Here's the drawing with two shaded views (mm, measured from the low corner). I have some questions. A direction names the side the tool comes from. Give positions to 0.01 mm unless a question says otherwise; leave off trailing zeros. Order: outer loops, then holes, each group sorted by start corner. A loop starts at its lowest first (then second) coordinate and runs counter-clockwise, first axis right, second up. Notation, with made-up numbers: M -4.75,18.5 L 13.25,18.5 A26 cw 13.25,35.5 Z; hole C 65.25,89 d11. An arc over 180 degrees is marked long. Use a Markdown table: item, result. Add a question column.
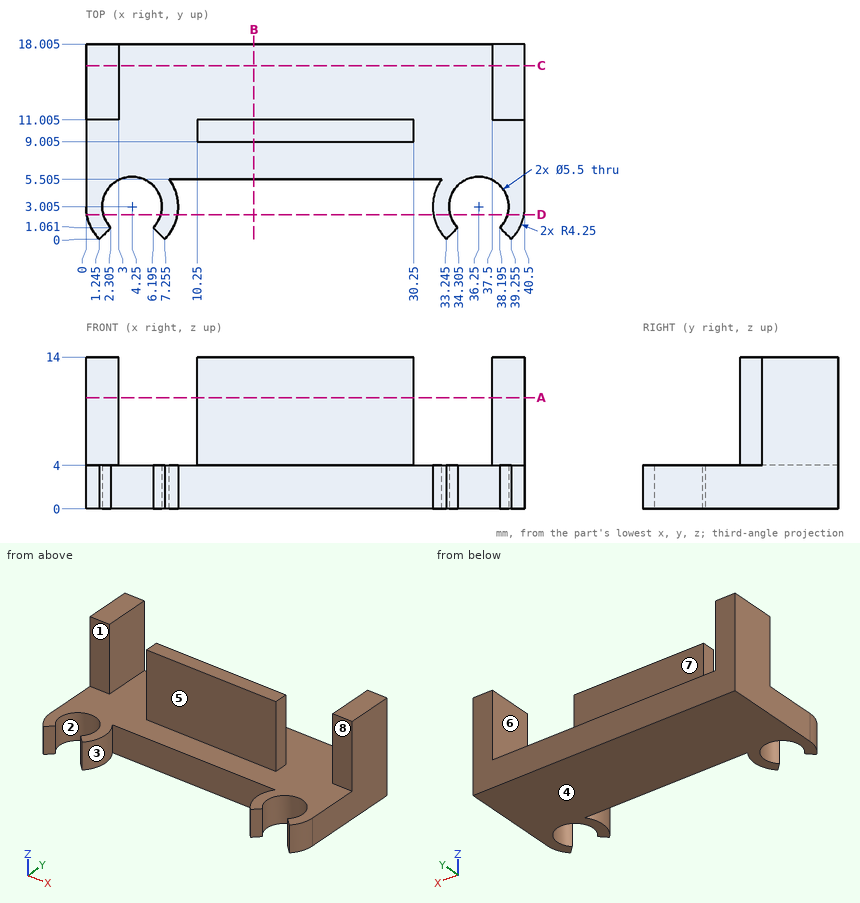
1. On a 3-axis mill with a long thin cutter (end or side, diameter ignored), from which of +Z, -Z, +X, -X, +Y, -Y can I reach the whole of each face in a straight line? I mean the marked faces 5, 6, 7 and 8. Say none if no direction works.
2. I need wall thicknesses on L1, parallel to X at y = 14.25, z = 4.25; L2, parallel to Y at x = 15, z = 10 (1 decimal); L3, parallel to Z at x = 2, y = 6.25. Which ranges of each line are inside material? Lowest first, please. Write a range as [from, to].
3. Will these pins go through, and if not, where does the flat tip stop? pin 1 (2 mm diameter, centred on x = 26, z = 3, fed in from -Y) (1 decimal); pin 2 (3 mm diameter, centred on x = 23, y = 13.5, fed in from +Z); pin 3 (4.5 mm diameter, centred on x = 36.25, y = 3.01, fed in from -Z); pin 4 (5 mm diameter, centred on x = 32.5, z = 11, fed in from -Y) (1 decimal).
4. We'd pull the mould along Y, two halves only. Please class the marked faces 1, 2, 3 and 4: +Y half, -Y half, draft (parallel to the pull), parting line (faces both ways), or undercut.
5. If we section it at B-B, the plane x = 15.5: List the corners of the cut face in (y, z) for me (1 decimal), then the cut area to 3 significant figures.
6. If we section it at A-A, the plane z = 10.25: State how many separate pieces and enclosed holes the cut face has.
7. If we section it at C-C, the plane y = 16: List the corners of the cut face in (x, z) for me.
8. If we section it at D-D, the plane y = 2.25: List the corners of the cut face in (x, z) for me (1 decimal), then the cut area to 3 significant figures.
Geometry results:
| question | item | result |
|---|---|---|
| 1 | face 5 | +Z, +X, -X, -Y |
| 1 | face 6 | +Z, +Y, -Y |
| 1 | face 7 | +Z, +Y |
| 1 | face 8 | +Z, +X, -Y |
| 2 | L1 | x = [0, 3], [37.5, 40.5] |
| 2 | L2 | y = [9, 11] |
| 2 | L3 | z = [0, 4] |
| 3 | pin 1 | stops at y = 5.5 |
| 3 | pin 2 | stops at z = 4 |
| 3 | pin 3 | passes through |
| 3 | pin 4 | stops at y = 9 |
| 4 | face 1 | -Y half |
| 4 | face 2 | undercut |
| 4 | face 3 | undercut |
| 4 | face 4 | draft |
| 5 | outline | M 5.5,0 L 18,0 L 18,4 L 11,4 L 11,14 L 9,14 L 9,4 L 5.5,4 Z |
| 5 | area | 70.0 mm^2 |
| 6 | separate pieces | 3 |
| 6 | enclosed holes | 0 |
| 7 | outline | M 0,0 L 40.5,0 L 40.5,14 L 37.5,14 L 37.5,4 L 3,4 L 3,14 L 0,14 Z |
| 8 | outline | M 0.1,0 L 1.6,0 L 1.6,4 L 0.1,4 Z; M 6.9,0 L 8.4,0 L 8.4,4 L 6.9,4 Z; M 32.1,0 L 33.6,0 L 33.6,4 L 32.1,4 Z; M 38.9,0 L 40.4,0 L 40.4,4 L 38.9,4 Z |
| 8 | area | 24.6 mm^2 |
